```python
from build123d import *

# Parameters (mm, degrees)
ESQUISSE1_R             = 0.85
BOSS_EXTRU_1_DEPTH      = 20
BOSS_EXTRU_2_DEPTH      = 5
ESQUISSE3_R             = 1.5
ENL_V_MAT_EXTRU_1_DEPTH = 47.234781527
CONG_1_R                = 1
CONG_2_R                = 3
CHANFREIN2_SIZE         = 2
ENL_V_MAT_EXTRU_2_DEPTH = 2
CHANFREIN3_SIZE         = 2
ENL_V_MAT_EXTRU_3_DEPTH = 47.234781527
CONG_3_R                = 5
CONG_4_R                = 3
BOSS_EXTRU_3_DEPTH      = 0.2


with BuildPart() as part:
    # Esquisse1 → Boss.-Extru.1 (new body)
    with BuildSketch(Plane.XY):
        Polygon((20, 25), (28, 25), (28, 0), (-28, 0), (-28, 25), (-20, 25), (-20, 5), (20, 5), align=None)
        with Locations((-24, 20)):
            Circle(ESQUISSE1_R, mode=Mode.SUBTRACT)
        with Locations((-24, 10)):
            Circle(ESQUISSE1_R, mode=Mode.SUBTRACT)
        with Locations(Location((24, 10, 0), (0, 0, 180))):
            Circle(ESQUISSE1_R, mode=Mode.SUBTRACT)
        with Locations(Location((24, 20, 0), (0, 0, 180))):
            Circle(ESQUISSE1_R, mode=Mode.SUBTRACT)
    extrude(amount=BOSS_EXTRU_1_DEPTH)

    # Esquisse2 → Boss.-Extru.2 (add)
    with BuildSketch(Plane(origin=(0, 5, 0), x_dir=(1, 0, 0), z_dir=(0, 1, 0))):
        Polygon((-25.117673753, 21.515226358), (28, 30.881305394), (28, -18.874598589), (-16.608913047, -26.740353539), align=None)
    extrude(amount=-BOSS_EXTRU_2_DEPTH)

    # Esquisse3 → Enlèv. mat.-Extru.1 (cut, through all)
    with BuildSketch(Plane(origin=(0, 5, 0), x_dir=(1, 0, 0), z_dir=(0, 1, 0))):
        with Locations(Location((-17.211954407, 16.307159752, 0), (0, 0, 270))):
            Circle(ESQUISSE3_R)
        with Locations(Location((6.128408145, -18.163515842, 0), (0, 0, 270))):
            Circle(ESQUISSE3_R)
        with Locations(Location((-10.960620011, -19.145919356, 0), (0, 0, 270))):
            Circle(ESQUISSE3_R)
    extrude(amount=-ENL_V_MAT_EXTRU_1_DEPTH, mode=Mode.SUBTRACT)

    # Congé1
    cong_1_edges = [part.edges().sort_by_distance(p)[0] for p in [
        (-20, 25, 10),
        (-20, 5, 10),
        (20, 5, 10),
        (20, 25, 10),
    ]]
    fillet(cong_1_edges, radius=CONG_1_R)

    # Congé2
    cong_2_edges = [part.edges().sort_by_distance(p)[0] for p in [
        (-28, 25, 10),
        (28, 25, 10),
    ]]
    fillet(cong_2_edges, radius=CONG_2_R)

    # Chanfrein2
    chanfrein2_edges = [part.edges().sort_by_distance(p)[0] for p in [
        (-10.960620011, 5, 17.645919356),
        (6.128408145, 5, 16.663515842),
    ]]
    chamfer(chanfrein2_edges, length=CHANFREIN2_SIZE)

    # Esquisse4 → Enlèv. mat.-Extru.2 (cut)
    with BuildSketch(Plane.XZ):
        Polygon((-48.23971452, 32.31771726), (0.015865378, 23.808956555), (-8.492895328, -24.446623343), (-56.748475225, -15.937862637), align=None)
    extrude(amount=-ENL_V_MAT_EXTRU_2_DEPTH, mode=Mode.SUBTRACT)

    # Chanfrein3
    chanfrein3_edges = [part.edges().sort_by_distance(p)[0] for p in [
        (-4.238514975, 2, -0.318833394),
    ]]
    chamfer(chanfrein3_edges, length=CHANFREIN3_SIZE - 0.0001)  # a hair under: the kernel refuses the full size

    # Esquisse5 → Enlèv. mat.-Extru.3 (cut, through all)
    with BuildSketch(Plane(origin=(0, 5, 0), x_dir=(1, 0, 0), z_dir=(0, 1, 0))):
        with BuildLine():
            Line((-28, -20), (-15.377035546, -20))
            ThreePointArc((-15.377035546, -20), (-13.722728197, -22.696262762), (-10.702454097, -23.636746706))
            Line((-10.702454097, -23.636746706), (6.649832575, -22.639209149))
            Line((6.649832575, -22.639209149), (6.649832575, -26.740353539))
            Line((6.649832575, -26.740353539), (-28, -26.740353539))
            Line((-28, -26.740353539), (-28, -20))
        make_face()
        Polygon((28, 30.881305394), (-21.886605112, 30.881305394), (8.994700282, 0), (28, 0), align=None)
    extrude(amount=-ENL_V_MAT_EXTRU_3_DEPTH, mode=Mode.SUBTRACT)

    # Congé3
    cong_3_edges = [part.edges().sort_by_distance(p)[0] for p in [
        (28, 0, 10),
        (-25.117673753, 3.5, -21.515226358),
        (-15.377035546, 3.5, 20),
        (-14.408791034, 3.5, -23.403491315),
        (8.994700282, 2.5, 0),
        (-21.32395885, 3.5, 0),
        (21.617531437, 2.5, 20),
    ]]
    fillet(cong_3_edges, radius=CONG_3_R)

    # Congé4
    cong_4_edges = [part.edges().sort_by_distance(p)[0] for p in [
        (-28, 2, 10),
    ]]
    fillet(cong_4_edges, radius=CONG_4_R)

    # Esquisse6 → Boss.-Extru.3 (add)
    with BuildSketch(Plane.XY.offset(20)):
        with BuildLine():
            Line((-28, 22), (-28, 5))
            ThreePointArc((-28, 5), (-27.121320344, 2.878679656), (-25, 2))
            Line((-25, 2), (-18.440348512, 2))
            Line((-18.440348512, 2), (-18.440348512, 5))
            Line((-18.440348512, 5), (-19, 5))
            ThreePointArc((-19, 5), (-19.707106781, 5.292893219), (-20, 6))
            Line((-20, 6), (-20, 24))
            ThreePointArc((-20, 24), (-20.292893219, 24.707106781), (-21, 25))
            Line((-21, 25), (-25, 25))
            ThreePointArc((-25, 25), (-27.121320344, 24.121320344), (-28, 22))
        make_face()
        with BuildLine():
            Line((19, 5), (22.054974755, 5))
            Line((22.054974755, 5), (22.054974755, 0))
            Line((22.054974755, 0), (23, 0))
            ThreePointArc((23, 0), (26.535533906, 1.464466094), (28, 5))
            Line((28, 5), (28, 22))
            ThreePointArc((28, 22), (27.121320344, 24.121320344), (25, 25))
            Line((25, 25), (21, 25))
            ThreePointArc((21, 25), (20.292893219, 24.707106781), (20, 24))
            Line((20, 24), (20, 6))
            ThreePointArc((20, 6), (19.707106781, 5.292893219), (19, 5))
        make_face()
    extrude(amount=-BOSS_EXTRU_3_DEPTH)


solid = part.part
```
The listing builds one solid part. Answer for the finished solid, in the listing's coordinates (mm). A direction names the side the tool comes from. Give positions to 0.01 mm unless a question says otherwise; leave off trailing zeros. Loops run counter-clockwise (first coordinate to the right, second up) from the corner with the lowest first, then second, coordinate; pieces in that order, holes last. Notation, with made-up numbers: (69, 6.5) - (78, 6.5) arc R11 ccw to (78, 13.5) - close; hole circle Ø7 at (80.5, 22). An arc over 180 degrees is marked (long way). Return JSON: item names as keys, results as strings. Group by question number.
1. Find section A-A (y = 20). Write down the section's boundary in (x, z).
2. Determine the mould class of faces 5 (the flat face through (24, 10, 19.8)), 6 (the flat face through (-23, 25, 10)), 7 (the flat face through (-0.22, 3.091, 23.034)) for opening direction Y: pulls with the +Y half, pulls with the -Y half, needs draft (parallel to the pull), parting line crosses it, or undercut.
3. Find section C-C (x = 24). Write down the section's boundary in (y, z), then the cut area to 3 significant figures.
4. Find section B-B (z = 1). State how many separate pieces and enclosed holes the cut face has, then the cut area to 3 significant figures.
5. Given pin 1 Ø2.5 at (x, z) = (-17.21, -16.31) entering from -Y; pin 2 Ø0.9 at (x, y) = (24.5, 20) entering from -Z; pin 3 Ø4 at (x, z) = (6.13, 18.16) entering from -Y; pin 4 Ø3 at (x, y) = (-22.5, 10.5) entering from +Z, each flat-ended and moving along its own axis, determine where each tip first touches the part or whether it passes through.
6. Which of the six approach directions +Z, -Z, +X, -X, +Y, -Y give full straight-line access (tool end or side, diameter ignored) to faces 1 (the flat face through (25, 13, 20)), 2 (the flat face through (-24, 10, 19.8)), 3 (the flat face through (-23.3, 3.5, -11.2)), 4 (the flat face through (-20, 15, 10))?
7. Straight lines are drawn through the part: line 1 (Y direction, x = -24, z = 7); line 2 (X direction, y = 20.5, z = 2); line 3 (X direction, y = 21, z = 4). For each, find the intervals that lie inside material, in ascending order. Write a range as [from, to].
Verdict:
{
 "1": {"outline": "(-28, 0) - (-24.85, 0) - (-24.85, 19.8) - (-23.15, 19.8) - (-23.15, 0) - (-20, 0) - (-20, 20) - (-28, 20) - close; (20, 0) - (23.15, 0) - (23.15, 19.8) - (24.85, 19.8) - (24.85, 0) - (28, 0) - (28, 20) - (20, 20) - close"},
 "2": {"face 5": "undercut", "face 6": "pulls with the +Y half", "face 7": "needs draft"},
 "3": {"outline": "(0.1, 0) - (9.15, 0) - (9.15, 19.8) - (10.85, 19.8) - (10.85, 0) - (19.15, 0) - (19.15, 19.8) - (20.85, 19.8) - (20.85, 0) - (25, 0) - (25, 20) - (0.1, 20) - close", "area": "431 mm^2"},
 "4": {"separate pieces": "1", "enclosed holes": "4", "area": "534 mm^2"},
 "5": {"pin 1": "passes through", "pin 2": "stops at z = 0", "pin 3": "stops at y = 0", "pin 4": "stops at z = 20"},
 "6": {"face 1": "+Z, +X, +Y", "face 2": "-Z", "face 3": "-X, +Y, -Y", "face 4": "+Z, -Z, +Y"},
 "7": {"line 1": "y = [2, 9.15], [10.85, 19.15], [20.85, 25]", "line 2": "x = [-28, -24.69], [-23.31, -20], [20, 23.31], [24.69, 28]", "line 3": "x = [-28, -20], [20, 28]"}
}
